Could you check a few things on this drawing? It's one solid part, dimensions in mm from its lowest x, y, z. Round coordinates to 2 decimals unless told otherwise and drop trailing zeros. Loops run counter-clockwise (first coordinate to the right, second up) from the corner with the lowest first, then second, coordinate; pieces in that order, holes last. Notation, with made-up numbers: M 7,31.25 L 59,31.25 A23 cw 59,58.25 Z; hole C 6.25,-30.75 d7. An arc over 180 degrees is marked long. Answer as a JSON object with one key per item and string values.
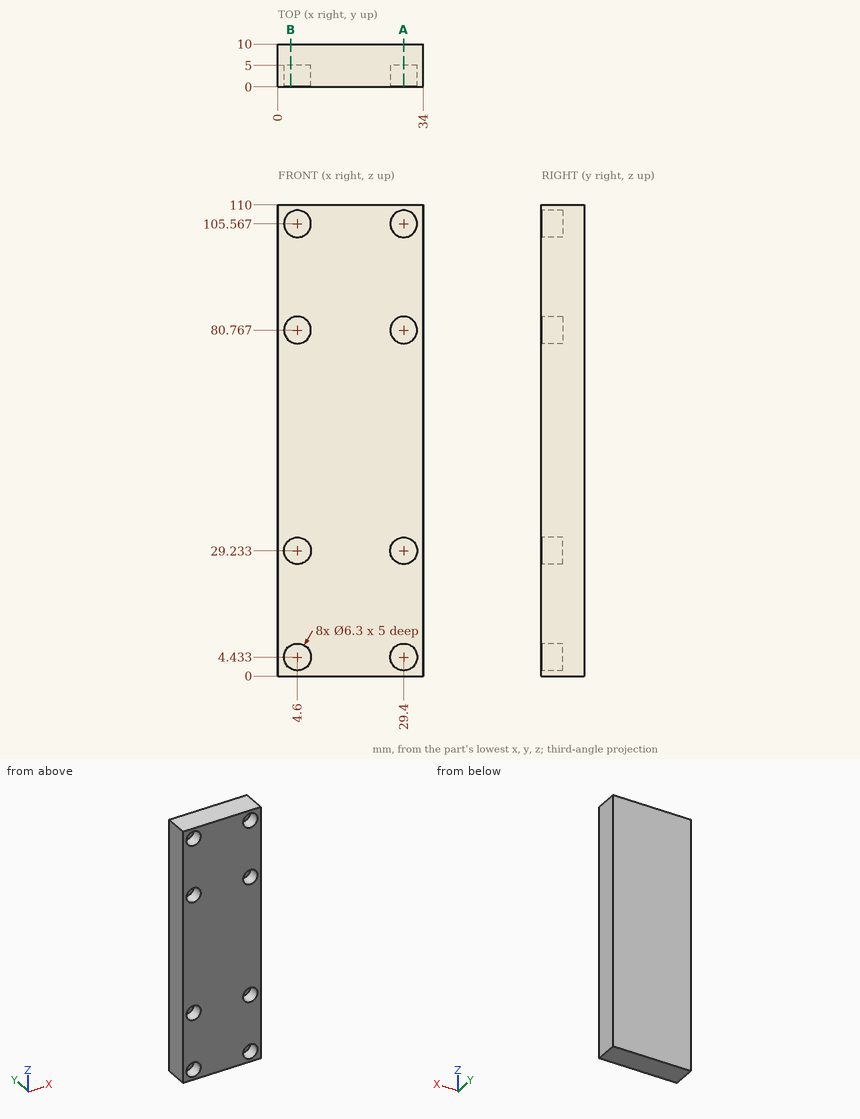
Item 1: Please list where these lines run through material, in increasing order: probe 1 along Z at (x, y) = (29.4, 3.3); probe 2 along Z at (x, y) = (28, 2.75) (1 decimal). Write a range as from..to.
Resolved:
{"probe 1": "0..1.28, 7.58..26.08, 32.38..77.62, 83.92..102.42, 108.72..110", "probe 2": "0..1.6, 7.3..26.4, 32.1..77.9, 83.6..102.7, 108.4..110"}
Item 2: I want a section at A-A, the plane x = 29.4. Please give me the cut outline in (y, z).
Resolved:
{"outline": "M 0,0 L 10,0 L 10,110 L 0,110 L 0,108.72 L 5,108.72 L 5,102.42 L 0,102.42 L 0,83.92 L 5,83.92 L 5,77.62 L 0,77.62 L 0,32.38 L 5,32.38 L 5,26.08 L 0,26.08 L 0,7.58 L 5,7.58 L 5,1.28 L 0,1.28 Z"}
Item 3: I want a section at B-B, the plane x = 3. Please give me the cut outline in (y, z).
Resolved:
{"outline": "M 0,0 L 10,0 L 10,110 L 0,110 L 0,108.28 L 5,108.28 L 5,102.85 L 0,102.85 L 0,83.48 L 5,83.48 L 5,78.05 L 0,78.05 L 0,31.95 L 5,31.95 L 5,26.52 L 0,26.52 L 0,7.15 L 5,7.15 L 5,1.72 L 0,1.72 Z"}
Item 4: I'm going to push a flat-ended pin straight in: pin 1 Ø1.9 at (x, z) = (5.5, 28.5) entering from -Y. Where does the tip first touch, or does it pass through?
Resolved:
{"pin 1": "y = 5"}
